Build history of the part. All positions in model axes, mm. A direction names the side the tool comes from. Round coordinates to 2 decimals unless told otherwise and drop trailing zeros. Order: outer loops, then holes, each group sorted by start corner. A loop starts at its lowest first (then second) coordinate and runs counter-clockwise, first axis right, second up. Notation, with made-up numbers: (6.25, 75) -> (25.25, 75) arc R14 cw to (25.25, 81) -> close; hole circle Ø2 at (39, 47). An arc over 180 degrees is marked (long way). Write item = value, one per line.
Autodesk Inventor part; units mm, degrees
ref_plane "YZ Plane" through (0, 0, 0) normal (1, 0, 0) x (0, 1, 0)
ref_plane "XZ Plane" through (0, 0, 0) normal (0, 1, 0) x (-1, 0, 0)
ref_plane "XY Plane" through (0, 0, 0) normal (0, 0, 1) x (1, 0, 0)
sketch "BASEsc" plane through (0, 0, 0) normal (0, 1, 0) x (-1, 0, 0)
  arc A0 (-30.7364, -0.0681) -> (-28.0904, 4.5242) centre (-30.3216, 2.7513) ccw
  arc A1 (-16.8277, 11.04) -> (-11.5277, 11.0446) centre (-14.1786, 12.0904) ccw
  arc A2 (-11.4967, -24.1586) -> (-16.7967, -24.1633) centre (-14.1458, -25.2091) ccw
  arc A3 (-0.2535, 4.5487) -> (2.4005, -0.0389) centre (1.9807, 2.7798) ccw
  arc A4 (-28.0709, -17.6674) -> (-30.7249, -13.0798) centre (-30.3051, -15.8984) ccw
  circle A5 centre (-14.1622, -6.5593) radius 17.8
  arc A6 (2.412, -13.0506) -> (-0.234, -17.6429) centre (1.9972, -15.87) ccw
  circle A7 centre (-55.7283, -6.3362) radius 17.9
  arc A8 (-58.3938, 11.2631) -> (-53.0938, 11.2678) centre (-55.7447, 12.3136) ccw
  arc A9 (-41.8196, 4.7719) -> (-39.1656, 0.1843) centre (-39.5854, 3.0029) ccw
  arc A10 (-72.3025, 0.1551) -> (-69.6565, 4.7474) centre (-71.8877, 2.9745) ccw
  arc A11 (-69.637, -17.4442) -> (-72.291, -12.8566) centre (-71.8712, -15.6753) ccw
  arc A12 (-53.0767, -24.0387) -> (-58.3776, -24.039) centre (-55.7271, -25.0859) ccw
  arc A13 (-39.1541, -12.8274) -> (-41.8001, -17.4197) centre (-39.569, -15.6468) ccw
  circle A14 centre (-101.6822, -6.2265) radius 18
  arc A15 (-99.0445, -24.0322) -> (-104.3463, -24.0282) centre (-101.6962, -25.0761) ccw
  arc A16 (-39.0717, -12.8911) -> (-41.7218, -17.4819) centre (-39.49, -15.71) ccw
  arc A17 (-41.7233, 4.8114) -> (-39.0725, 0.2209) centre (-39.4912, 3.0397) ccw
  arc A18 (-58.3799, 11.3664) -> (-53.079, 11.3667) centre (-55.7295, 12.4135) ccw
  arc A19 (-72.3849, 0.2188) -> (-69.7348, 4.8096) centre (-71.9666, 3.0377) ccw
  arc A20 (-69.7334, -17.4837) -> (-72.3841, -12.8932) centre (-71.9654, -15.7121) ccw
  circle A21 centre (43.1966, -7.3809) radius 17.7
  arc A22 (45.8761, -24.8769) -> (40.5769, -24.886) centre (43.2283, -25.9306) ccw
  circle A23 centre (45.2732, 42.9601) radius 17.7
  arc A24 (47.7889, 25.4398) -> (42.6535, 25.455) centre (45.2175, 24.2112) ccw
  arc A25 (-51.2492, 27.6525) -> (-56.3871, 27.6758) centre (-53.8237, 26.4307) ccw
  circle A26 centre (-53.7378, 45.3786) radius 17.9
  arc A27 (-84.9432, -12.845) -> (-87.5975, -17.4345) centre (-85.365, -15.6634) ccw
  arc A28 (-87.5809, 4.9607) -> (-84.9334, 0.3672) centre (-85.351, 3.1862) ccw
  arc A29 (-104.3199, 11.5792) -> (-99.0181, 11.5753) centre (-101.6682, 12.6231) ccw
  arc A30 (-118.4212, 0.3921) -> (-115.7669, 4.9816) centre (-117.9994, 3.2104) ccw
  arc A31 (-115.7835, -17.4136) -> (-118.431, -12.8202) centre (-118.0134, -15.6392) ccw
  arc A32 (-37.1422, 38.6707) -> (-39.7313, 34.2328) centre (-37.3714, 35.8302) ccw
  arc A33 (-39.6308, 56.3969) -> (-37.082, 51.9357) centre (-37.2854, 54.7782) ccw
  arc A34 (-56.2264, 63.1048) -> (-51.0885, 63.0815) centre (-53.6518, 64.3265) ccw
  arc A35 (-70.3334, 52.0865) -> (-67.7443, 56.5244) centre (-70.1042, 54.927) ccw
  arc A36 (-67.8448, 34.3603) -> (-70.3936, 38.8215) centre (-70.1901, 35.9791) ccw
  arc A37 (61.7041, 36.3785) -> (59.1232, 31.9388) centre (61.4824, 33.5374) ccw
  arc A38 (59.1885, 53.8989) -> (61.7429, 49.4439) centre (61.5381, 52.2863) ccw
  arc A39 (42.7576, 60.4804) -> (47.8929, 60.4652) centre (45.3289, 61.7089) ccw
  arc A40 (28.8424, 49.5417) -> (31.4233, 53.9813) centre (29.0641, 52.3828) ccw
  arc A41 (31.358, 32.0213) -> (28.8036, 36.4763) centre (29.0084, 33.6339) ccw
  arc A42 (59.6883, -13.8084) -> (57.0466, -18.4022) centre (59.2769, -16.6283) ccw
  arc A43 (57.0088, 3.6876) -> (59.6663, -0.8971) centre (59.2452, 1.9214) ccw
  arc A44 (40.5171, 10.1151) -> (45.8163, 10.1242) centre (43.1649, 11.1688) ccw
  arc A45 (26.7049, -0.9534) -> (29.3466, 3.6404) centre (27.1162, 1.8665) ccw
  arc A46 (29.3843, -18.4494) -> (26.7269, -13.8647) centre (27.1479, -16.6832) ccw
  line L0 (39.5339, -31.8115) -> (-97.6905, -31.8115)
  line L1 (-132.6905, 3.1885) -> (-132.6905, 34.7246)
  line L2 (-76.3868, 69.7246) -> (-21.7967, 69.7246)
  line L3 (74.5339, 34.7246) -> (74.5339, 3.1885)
  arc A47 (34.5339, -31.8115) -> (74.5339, 8.1885) centre (34.5339, 8.1885) ccw
  arc A48 (74.5339, 34.7246) -> (39.5339, 69.7246) centre (39.5339, 34.7246) ccw
  arc A49 (39.5339, -31.8115) -> (74.5339, 3.1885) centre (39.5339, 3.1885) ccw
  arc A50 (-132.6905, 3.1885) -> (-97.6905, -31.8115) centre (-97.6905, 3.1885) ccw
  arc A51 (-97.6905, 69.7246) -> (-132.6905, 34.7246) centre (-97.6905, 34.7246) ccw
  line L4 (-86.3868, 24.2112) -> (-132.6905, 24.2112)
  line L5 (-132.6905, 24.2112) -> (-132.6905, 69.7246)
  line L6 (-132.6905, 69.7246) -> (-81.3868, 69.7246)
  line L7 (-81.3868, 64.7246) -> (-81.3868, 29.2112)
  line L8 (14.5191, 69.7246) -> (-16.7967, 69.7246)
  line L9 (-16.7967, 64.7246) -> (-16.7967, 23.9565)
  line L10 (-11.7967, 18.9565) -> (9.5191, 18.9565)
  line L11 (14.5191, 23.9565) -> (14.5191, 69.7246)
  arc A52 (9.5191, 18.9565) -> (14.5191, 23.9565) centre (9.5191, 23.9565) ccw
  arc A53 (-16.7967, 23.9565) -> (-11.7967, 18.9565) centre (-11.7967, 23.9565) ccw
  arc A54 (-86.3868, 24.2112) -> (-81.3868, 29.2112) centre (-86.3868, 29.2112) ccw
  arc A55 (-76.3868, 69.7246) -> (-81.3868, 64.7246) centre (-76.3868, 64.7246) ccw
  arc A56 (-16.7967, 64.7246) -> (-21.7967, 69.7246) centre (-21.7967, 64.7246) ccw
  line L12 (39.5339, 69.7246) -> (-21.7967, 69.7246)
  point P0 (0, 0)
  point P1 (-14.1467, -24.3593)
  point P2 (-27.8531, 1.3272)
  point P3 (-14.1777, 9.2407)
  point P4 (-14.1467, -22.3593)
  point P5 (-0.4868, 1.3541)
  point P6 (-27.8376, -14.4728)
  point P7 (-0.4712, -14.4459)
  point P8 (-41.5661, 0.2232)
  point P9 (-55.7127, -24.2361)
  point P10 (-55.7438, 9.4638)
  point P11 (-42.0529, 1.5773)
  point P12 (-69.4193, 1.5504)
  point P13 (-69.4038, -14.2496)
  point P14 (-55.7127, -22.2361)
  point P15 (-42.0374, -14.2227)
  point P16 (-87.52, 0.3329)
  point P17 (-101.6665, -24.2265)
  point P18 (-101.6977, 9.5735)
  point P19 (-88.0068, 1.6869)
  point P20 (-115.3732, 1.6601)
  point P21 (-115.3576, -14.1399)
  point P22 (-101.6665, -22.2265)
  point P23 (-87.9913, -14.1131)
  point P24 (-41.9507, -14.2726)
  point P25 (-41.9663, 1.6273)
  point P26 (-55.7439, 9.5638)
  point P27 (-69.5059, 1.6003)
  point P28 (-69.4903, -14.2997)
  point P29 (57.3588, -0.8216)
  point P30 (29.5211, -15.2943)
  point P31 (56.872, 0.5325)
  point P32 (43.212, -25.0809)
  point P33 (29.5056, 0.5057)
  point P34 (43.1811, 8.4191)
  point P35 (56.8875, -15.2675)
  point P36 (43.212, -23.0809)
  point P37 (59.4354, 49.5194)
  point P38 (31.5978, 35.0467)
  point P39 (58.9487, 50.8735)
  point P40 (45.2887, 25.2601)
  point P41 (31.5823, 50.8467)
  point P42 (45.2577, 58.7601)
  point P43 (58.9642, 35.0735)
  point P44 (45.2887, 27.0601)
  point P45 (-40.0468, 37.492)
  point P46 (-39.5756, 51.9379)
  point P47 (-40.0623, 53.292)
  point P48 (-53.7222, 29.2786)
  point P49 (-53.7222, 27.4786)
  point P50 (-53.7533, 61.1786)
  point P51 (-67.4287, 53.2652)
  point P52 (-67.4132, 37.4652)
  point P53 (-87.818, -14.2129)
  point P54 (-87.8336, 1.7871)
  point P55 (-101.6979, 9.7735)
  point P56 (-115.5464, 1.7599)
  point P57 (-115.5308, -14.2401)
  point P58 (-39.787, 37.3421)
  point P59 (-39.8026, 53.4421)
  point P60 (-53.7534, 61.4786)
  point P61 (-67.6886, 53.4151)
  point P62 (-67.673, 37.3151)
  point P63 (59.0507, 35.0234)
  point P64 (59.0353, 50.9234)
  point P65 (45.2578, 58.8601)
  point P66 (31.4957, 50.8967)
  point P67 (31.5111, 34.9967)
  point P68 (56.8009, -15.2175)
  point P69 (56.7855, 0.4824)
  point P70 (43.1812, 8.3191)
  point P71 (29.5923, 0.4557)
  point P72 (29.6077, -15.2442)
  point P73 (-97.6905, 69.7246)
  point P74 (-16.7967, 69.7246)
  point P75 (-67.8448, 34.3603)
  point P76 (-39.7313, 34.2328)
  point P77 (-37.1422, 38.6707)
  point P78 (-37.082, 51.9357)
  point P79 (-51.0885, 63.0815)
  point P80 (-67.7443, 56.5244)
  point P81 (-70.3334, 52.0865)
  point P82 (-118.431, -12.8202)
  point P83 (-115.7835, -17.4136)
  point P84 (-87.5975, -17.4345)
  point P85 (-84.9334, 0.3672)
  point P86 (-87.5809, 4.9607)
  point P87 (-104.3199, 11.5792)
  point P88 (-115.7669, 4.9816)
  point P89 (-118.4212, 0.3921)
  point P90 (-72.3841, -12.8932)
  point P91 (-39.0725, 0.2209)
  point P92 (-41.7233, 4.8114)
  point P93 (-53.079, 11.3667)
  point P94 (-58.3799, 11.3664)
  point P95 (-69.7348, 4.8096)
  point P96 (-72.3849, 0.2188)
  point P97 (-0.234, -17.6429)
  point P98 (2.412, -13.0506)
  point P99 (2.4005, -0.0389)
  point P100 (-0.2535, 4.5487)
  point P101 (-11.5277, 11.0446)
  point P102 (-16.8277, 11.04)
  point P103 (-28.0904, 4.5242)
  point P104 (-30.7364, -0.0681)
  point P105 (-28.0709, -17.6674)
  point P106 (29.3843, -18.4494)
  point P107 (59.6883, -13.8084)
  point P108 (59.6663, -0.8971)
  point P109 (57.0088, 3.6876)
  point P110 (40.5171, 10.1151)
  point P111 (29.3466, 3.6404)
  point P112 (26.7049, -0.9534)
  point P113 (47.8929, 60.4652)
  point P114 (31.4233, 53.9813)
  point P115 (28.8424, 49.5417)
  dimension "d0" = 35.6
  dimension "d1" = 2
  dimension "d2" = 35.8
  dimension "d3" = 2
  dimension "d4" = 36
  dimension "d5" = 2
  dimension "d8" = 360
  dimension "d10" = 35.4
  dimension "d11" = 2
  dimension "d12" = 35.4
  dimension "d13" = 1.8
  dimension "d14" = 35.8
  dimension "d15" = 1.8
  dimension "d18" = 360
  dimension "d22" = 360
  dimension "d26" = 360
  dimension "d30" = 360
  dimension "d32" = 40
  dimension "d33" = 35
  dimension "d34" = 35
  dimension "d35" = 35
  dimension "d36" = 5
extrude "押し出し1" add sketch "BASEsc" against normal blind 2.5 contours A5 A0 | A0 A5 A1 A3 A6 A2 A4 | A4 A5 | A5 A1 | A2 A5 | A5 A3 | A6 A5 | A7 A16 A12 A20 A19 A18 A17 | A17 A7 | A7 A16 | A18 A7 | A7 A12 | A19 A7 | A7 A20 | A14 A27 A15 A31 A30 A29 A28 | A28 A14 | A14 A27 | A29 A14 | A14 A15 | A30 A14 | A14 A31 | A21 A42 A22 A46 A45 A44 A43 | A43 A21 | A21 A42 | A44 A21 | A21 A22 | A45 A21 | A21 A46 | A23 A37 A24 A41 A40 A39 A38 | A38 A23 | A23 A37 | A39 A23 | A23 A24 | A40 A23 | A23 A41 | A26 A25 | A25 A26 A36 A35 A34 A33 A32 | A32 A26 | A26 A36 | A26 A35 | A33 A26 | A26 A34 | L5 L6 A51 | L0 A47 L3 A49 | L0 A50 L1 L4 A54 L7 A55 L2 A56 L9 A53 L10 A52 L11 L12 A48 L3 A47 | L11 A52 L10 A53 L9 A56 L12 L8
extrude "押し出し2" cut sketch "BASEsc" against normal through all contours A0 A5 A1 A3 A6 A2 A4 | A7 A16 A12 A20 A19 A18 A17 | A14 A27 A15 A31 A30 A29 A28 | A21 A42 A22 A46 A45 A44 A43 | A23 A37 A24 A41 A40 A39 A38 | A25 A26 A36 A35 A34 A33 A32
extrude "押し出し3" cut sketch "BASEsc" against normal blind 10 contours L5 L6 A51 | L11 A52 L10 A53 L9 A56 L12 L8
fillet "フィレット1" radius 25 1 edges at (132.6905, -1.25, 24.2112)
equation "\"BendRadius\" = Thickness"
equation "\"BendReliefWidth\" = Thickness"
equation "\"BendReliefDepth\" = 0.5 * Thickness"
equation "\"CornerReliefSize\" = 4 * Thickness"
equation "\"MinimumRemnant\" = 2 * Thickness"
equation "\"TransitionRadius\" = BendRadius"
equation "\"JacobiRadiusSize\" = BendRadius"
equation "\"GapSize\" = Thickness"
properties part number "template"
Q1. Flat gauge pins, fed straight in: pin 1 (1.2 mm diameter, centred on y = -1, z = 36, fed in from +X); pin 2 (0.8 mm diameter, centred on x = 98.5, y = -1.5, fed in from +Z); pin 3 (1.5 mm diameter, centred on y = -2, z = 22, fed in from +X). Where does each tip first touch, or does it go through?
Check values:
pin_1 = 81.39
pin_2 = 24.21
pin_3 = 118.67
Q2. Probe probe 1 along X at (y, z) = (-0.75, 7.5); probe 2 along Z at (x, y) = (-53, -0.25); probe 3 along Z at (x, y) = (52, -0.75). List the from-to ranges inside material, lowest first.
Check values:
probe_1 = -74.53 to -52.78, -33.61 to 3.25, 25.08 to 44.37, 67.08 to 90.04, 113.33 to 130.45
probe_2 = -29.12 to -22.12, 7.36 to 27.04, 58.88 to 67.03
probe_3 = -31.81 to -23.84, 11.17 to 28.62, 62 to 69.72
Q3. Cut at B-B, the plane z = 47. List the corners of the cut face in (x, y), and give its area (3 significant figures).
Check values:
outline = (-72.31, -2.5) -> (-62.51, -2.5) -> (-62.51, 0) -> (-72.31, 0) -> close; (-28.04, -2.5) -> (-14.52, -2.5) -> (-14.52, 0) -> (-28.04, 0) -> close; (16.8, -2.5) -> (35.91, -2.5) -> (35.91, 0) -> (16.8, 0) -> close; (71.56, -2.5) -> (81.39, -2.5) -> (81.39, 0) -> (71.56, 0) -> close
area = 131 mm²
Q4. Mould opens along Z. For faces 1 (the face through (22.995, -1.232, 8.895)), 2 (the face through (92.59, -1.23, 9.31)), 3 (the face through (-64.01, -1.23, -21.83)), 4 (the face through (-13.016, -1.232, 20.382)) say: released by +Z, released by -Z, zero draft, split by the parting line, or undercut.
Check values:
face_1 = undercut
face_2 = undercut
face_3 = released by -Z
face_4 = released by +Z
Q5. Which spindle directions (+Z, -Z, +X, -X, +Y, -Y) get a long thin tool onto all of the face, cutting with end or side? Do faces 5 (the face through (18.2, -1.2, 68.2)), 6 (the face through (-51.99, -1.23, -22.74)), 7 (the face through (-64.553, -1.232, 59.2)). Say none if no direction does.
Check values:
face_5 = +Z, +Y, -Y
face_6 = +Y, -Y
face_7 = +Z, -X, +Y, -Y
Q6. Cut at A-A, the plane x = 94. List the corners of the cut face in (y, z).
Check values:
outline = (-2.5, -31.81) -> (0, -31.81) -> (0, -22.5) -> (-2.5, -22.5) -> close; (-2.5, 10.05) -> (0, 10.05) -> (0, 24.21) -> (-2.5, 24.21) -> close
Q7. Cut at C-C, the plane y = -2.1. Give the number of separate pieces and of enclosed holes in the cut face, and give its area (3 significant figures).
Check values:
separate_pieces = 1
enclosed_holes = 6
area = 10,400 mm²
